```python
from build123d import *

# Parameters (mm, degrees)
SKETCH2_W           = 292
SKETCH2_H           = 160
BOSS_EXTRUDE1_DEPTH = 3
BOSS_EXTRUDE2_DEPTH = 3
BOSS_EXTRUDE3_START = -35
BOSS_EXTRUDE3_DEPTH = 55
SKETCH5_R           = 1.9
BOSS_EXTRUDE4_DEPTH = 5
BOSS_EXTRUDE5_START = 35
BOSS_EXTRUDE5_DEPTH = 35
SKETCH5_5_R         = 1.9
CUT_EXTRUDE1_DEPTH  = 309.76121842
SKETCH6_R           = 1.9
SKETCH6_W           = 6.2
SKETCH6_H           = 14.6
CUT_EXTRUDE2_DEPTH  = 225.15461182
SKETCH7_R           = 1.75
CUT_EXTRUDE3_DEPTH  = 225.15461182
BOSS_EXTRUDE6_DEPTH = 3
BOSS_EXTRUDE7_DEPTH = 21
SKETCH8_3_W         = 32
SKETCH8_3_H         = 38
CUT_EXTRUDE4_DEPTH  = 221.209195993


with BuildPart() as part:
    # Sketch2 → Boss-Extrude1 (new body)
    with BuildSketch(Plane(origin=(0, 0, 0), x_dir=(1, 0, 0), z_dir=(0, 1, 0))):
        with Locations((0, 80)):
            Rectangle(SKETCH2_W, SKETCH2_H)
    extrude(amount=BOSS_EXTRUDE1_DEPTH)

    # Sketch3 → Boss-Extrude2 (add)
    with BuildSketch(Plane(origin=(0, 3, 0), x_dir=(1, 0, 0), z_dir=(0, 1, 0))):
        with BuildLine():
            ThreePointArc((-49.25, -30.5), (-40.316756826, -8.933243174), (-18.75, 0))
            Line((-18.75, 0), (-146, 0))
            Line((-146, 0), (-146, -30.5))
            Line((-146, -30.5), (-49.25, -30.5))
        make_face()
        with BuildLine():
            Line((146, -30.5), (146, 0))
            Line((146, 0), (18.75, 0))
            ThreePointArc((18.75, 0), (40.316756826, -8.933243174), (49.25, -30.5))
            Line((49.25, -30.5), (146, -30.5))
        make_face()
    extrude(amount=-BOSS_EXTRUDE2_DEPTH)

    # Sketch4 → Boss-Extrude3 (add)
    with BuildSketch(Plane(origin=(146, 0, 0), x_dir=(0, 0, -1), z_dir=(1, 0, 0)).offset(BOSS_EXTRUDE3_START)):
        with BuildLine():
            Line((10.8, 21.7), (10.8, 3))
            Line((10.8, 3), (32.499999845, 3))
            ThreePointArc((32.499999845, 3), (19.277103137, 8.477103246), (13.8, 21.7))
            Line((13.8, 21.7), (10.8, 21.7))
        make_face()
        with BuildLine():
            ThreePointArc((51.2, 21.7), (45.722896754, 8.477103137), (32.499999845, 3))
            Line((32.499999845, 3), (54.2, 3))
            Line((54.2, 3), (54.2, 21.7))
            Line((54.2, 21.7), (51.2, 21.7))
        make_face()
    boss_extrude3 = extrude(amount=-BOSS_EXTRUDE3_DEPTH)

    # Sketch5 → Boss-Extrude4 (add)
    # profile 1 of 3: a face of its own
    with BuildSketch(Plane(origin=(111, 0, 0), x_dir=(0, 0, -1), z_dir=(1, 0, 0))):
        with BuildLine():
            Line((-4.5, 21.7), (-4.5, 0))
            Line((-4.5, 0), (69.5, 0))
            Line((69.5, 0), (69.5, 21.7))
            ThreePointArc((69.5, 21.7), (32.5, 58.7), (-4.5, 21.7))
        make_face()
        with Locations((24.875, 8.493112592)):
            Circle(SKETCH5_R, mode=Mode.SUBTRACT)
        with Locations((17.25, 21.7)):
            Circle(SKETCH5_R, mode=Mode.SUBTRACT)
        with Locations((40.125, 8.493112592)):
            Circle(SKETCH5_R, mode=Mode.SUBTRACT)
        with BuildLine():
            ThreePointArc((32.5, 3), (45.722896808, 8.477103192), (51.2, 21.7))
            Line((51.2, 21.7), (54.2, 21.7))
            Line((54.2, 21.7), (54.2, 3))
            Line((54.2, 3), (32.5, 3))
        make_face(mode=Mode.SUBTRACT)
        with BuildLine():
            ThreePointArc((26.3, 23.2), (32.5, 29.4), (38.7, 23.2))
            Line((38.7, 23.2), (38.7, 20.2))
            ThreePointArc((38.7, 20.2), (32.5, 14), (26.3, 20.2))
            Line((26.3, 20.2), (26.3, 23.2))
        make_face(mode=Mode.SUBTRACT)
        with Locations((47.75, 21.7)):
            Circle(SKETCH5_R, mode=Mode.SUBTRACT)
        with Locations((24.875, 34.906887408)):
            Circle(SKETCH5_R, mode=Mode.SUBTRACT)
        with Locations((40.125, 34.906887408)):
            Circle(SKETCH5_R, mode=Mode.SUBTRACT)
    # profile 2 of 3: a face of its own
    with BuildSketch(Plane(origin=(111, 0, 0), x_dir=(0, 0, -1), z_dir=(1, 0, 0))):
        with BuildLine():
            Line((-6.5, 0), (-4.5, 0))
            Line((-4.5, 0), (-4.5, 21.7))
            ThreePointArc((-4.5, 21.7), (32.5, 58.7), (69.5, 21.7))
            Line((69.5, 21.7), (69.5, 0))
            Line((69.5, 0), (71.5, 0))
            Line((71.5, 0), (71.5, 21.7))
            ThreePointArc((71.5, 21.7), (32.5, 60.7), (-6.5, 21.7))
            Line((-6.5, 21.7), (-6.5, 0))
        make_face()
    # profile 3 of 3: a face of its own
    with BuildSketch(Plane(origin=(111, 0, 0), x_dir=(0, 0, -1), z_dir=(1, 0, 0))):
        with BuildLine():
            Line((54.2, 21.7), (51.2, 21.7))
            ThreePointArc((51.2, 21.7), (45.722896808, 8.477103192), (32.5, 3))
            Line((32.5, 3), (54.2, 3))
            Line((54.2, 3), (54.2, 21.7))
        make_face()
    boss_extrude4 = extrude(amount=-BOSS_EXTRUDE4_DEPTH)

    # Sketch5<4> → Boss-Extrude5 (add)
    with BuildSketch(Plane(origin=(111, 0, 0), x_dir=(0, 0, -1), z_dir=(1, 0, 0)).offset(BOSS_EXTRUDE5_START)):
        with BuildLine():
            Line((-6.5, 0), (-4.5, 0))
            Line((-4.5, 0), (-4.5, 21.7))
            ThreePointArc((-4.5, 21.7), (32.5, 58.7), (69.5, 21.7))
            Line((69.5, 21.7), (69.5, 0))
            Line((69.5, 0), (71.5, 0))
            Line((71.5, 0), (71.5, 21.7))
            ThreePointArc((71.5, 21.7), (32.5, 60.7), (-6.5, 21.7))
            Line((-6.5, 21.7), (-6.5, 0))
        make_face()
    boss_extrude5 = extrude(amount=-BOSS_EXTRUDE5_DEPTH)

    # Sketch5<5> → Cut-Extrude1 (cut, through all)
    # profile 1 of 2: a face of its own
    with BuildSketch(Plane(origin=(111, 0, 0), x_dir=(0, 0, -1), z_dir=(1, 0, 0))):
        with BuildLine():
            Line((-4.5, 21.7), (-4.5, 0))
            Line((-4.5, 0), (69.5, 0))
            Line((69.5, 0), (69.5, 21.7))
            ThreePointArc((69.5, 21.7), (32.5, 58.7), (-4.5, 21.7))
        make_face()
        with Locations((24.875, 8.493112592)):
            Circle(SKETCH5_5_R, mode=Mode.SUBTRACT)
        with Locations((17.25, 21.7)):
            Circle(SKETCH5_5_R, mode=Mode.SUBTRACT)
        with Locations((40.125, 8.493112592)):
            Circle(SKETCH5_5_R, mode=Mode.SUBTRACT)
        with BuildLine():
            ThreePointArc((32.5, 3), (45.722896808, 8.477103192), (51.2, 21.7))
            Line((51.2, 21.7), (54.2, 21.7))
            Line((54.2, 21.7), (54.2, 3))
            Line((54.2, 3), (32.5, 3))
        make_face(mode=Mode.SUBTRACT)
        with BuildLine():
            ThreePointArc((26.3, 23.2), (32.5, 29.4), (38.7, 23.2))
            Line((38.7, 23.2), (38.7, 20.2))
            ThreePointArc((38.7, 20.2), (32.5, 14), (26.3, 20.2))
            Line((26.3, 20.2), (26.3, 23.2))
        make_face(mode=Mode.SUBTRACT)
        with Locations((47.75, 21.7)):
            Circle(SKETCH5_5_R, mode=Mode.SUBTRACT)
        with Locations((24.875, 34.906887408)):
            Circle(SKETCH5_5_R, mode=Mode.SUBTRACT)
        with Locations((40.125, 34.906887408)):
            Circle(SKETCH5_5_R, mode=Mode.SUBTRACT)
    # profile 2 of 2: a face of its own
    with BuildSketch(Plane(origin=(111, 0, 0), x_dir=(0, 0, -1), z_dir=(1, 0, 0))):
        with BuildLine():
            Line((54.2, 21.7), (51.2, 21.7))
            ThreePointArc((51.2, 21.7), (45.722896808, 8.477103192), (32.5, 3))
            Line((32.5, 3), (54.2, 3))
            Line((54.2, 3), (54.2, 21.7))
        make_face()
    cut_extrude1 = extrude(amount=CUT_EXTRUDE1_DEPTH, mode=Mode.SUBTRACT)

    # Sketch6 → Cut-Extrude2 (cut, through all)
    with BuildSketch(Plane(origin=(0, 3, 0), x_dir=(1, 0, 0), z_dir=(0, 1, 0))):
        with Locations(Location((120.3, -18.5, 0), (0, 0, 270))):
            Circle(SKETCH6_R)
        with Locations((140.9, -18.5)):
            Rectangle(SKETCH6_W, SKETCH6_H)
    cut_extrude2 = extrude(amount=-CUT_EXTRUDE2_DEPTH, mode=Mode.SUBTRACT)

    # Mirror1: Boss-Extrude3, Boss-Extrude4, Boss-Extrude5, Cut-Extrude1, Cut-Extrude2 across plane
    add(boss_extrude3.mirror(Plane(origin=(0, 0, 0), x_dir=(0, 0, 1), z_dir=(1, 0, 0))))
    add(boss_extrude4.mirror(Plane(origin=(0, 0, 0), x_dir=(0, 0, 1), z_dir=(1, 0, 0))))
    add(boss_extrude5.mirror(Plane(origin=(0, 0, 0), x_dir=(0, 0, 1), z_dir=(1, 0, 0))))
    add(cut_extrude1.mirror(Plane(origin=(0, 0, 0), x_dir=(0, 0, 1), z_dir=(1, 0, 0))), mode=Mode.SUBTRACT)
    add(cut_extrude2.mirror(Plane(origin=(0, 0, 0), x_dir=(0, 0, 1), z_dir=(1, 0, 0))), mode=Mode.SUBTRACT)

    # Sketch7 → Cut-Extrude3 (cut, through all)
    with BuildSketch(Plane(origin=(0, 3, 0), x_dir=(1, 0, 0), z_dir=(0, 1, 0))):
        with Locations(Location((-18, 14.5, 0), (0, 0, 270))):
            Circle(SKETCH7_R)
        with Locations(Location((18, 14.5, 0), (0, 0, 270))):
            Circle(SKETCH7_R)
        with Locations(Location((18, 50.5, 0), (0, 0, 270))):
            Circle(SKETCH7_R)
        with Locations(Location((-18, 50.5, 0), (0, 0, 270))):
            Circle(SKETCH7_R)
    extrude(amount=-CUT_EXTRUDE3_DEPTH, mode=Mode.SUBTRACT)



with BuildPart() as body_2:
    # Sketch8 → Boss-Extrude6 (new body)
    with BuildSketch(Plane(origin=(0, 21, 0), x_dir=(1, 0, 0), z_dir=(0, 1, 0))):
        with BuildLine():
            Line((-35, 141), (-35, 160))
            Line((-35, 160), (35, 160))
            Line((35, 160), (35, 141))
            ThreePointArc((35, 141), (0, 106), (-35, 141))
        make_face()
    extrude(amount=BOSS_EXTRUDE6_DEPTH)


with BuildPart() as part_1:
    add(part.part)

    add(body_2.part)  # Boss-Extrude7 merges body 2
    # Sketch10 → Boss-Extrude7 (add)
    with BuildSketch(Plane(origin=(0, 24, 0), x_dir=(1, 0, 0), z_dir=(0, 1, 0))):
        with BuildLine():
            Line((-38, 160), (-38, 141))
            ThreePointArc((-38, 141), (0, 103), (38, 141))
            Line((38, 141), (38, 160))
            Line((38, 160), (35, 160))
            Line((35, 160), (35, 141))
            ThreePointArc((35, 141), (0, 106), (-35, 141))
            Line((-35, 141), (-35, 160))
            Line((-35, 160), (-38, 160))
        make_face()
    extrude(amount=-BOSS_EXTRUDE7_DEPTH)

    # Sketch8<3> → Cut-Extrude4 (cut, through all)
    with BuildSketch(Plane(origin=(0, 21, 0), x_dir=(1, 0, 0), z_dir=(0, 1, 0))):
        with Locations((0, 141)):
            Rectangle(SKETCH8_3_W, SKETCH8_3_H)
        with BuildLine():
            Line((-16, 122), (-16, 160))
            Line((-16, 160), (-35, 160))
            Line((-35, 160), (-35, 141))
            ThreePointArc((-35, 141), (0, 106), (35, 141))
            Line((35, 141), (35, 160))
            Line((35, 160), (16, 160))
            Line((16, 160), (16, 122))
            Line((16, 122), (-16, 122))
        make_face()
    extrude(amount=-CUT_EXTRUDE4_DEPTH, mode=Mode.SUBTRACT)


solid = part_1.part
```
The model under review builds one solid part; all positions refer to its coordinate system, in mm. A direction names the side the tool comes from. Give positions to 0.01 mm unless a question says otherwise; leave off trailing zeros. Order: outer loops, then holes, each group sorted by start corner. A loop starts at its lowest first (then second) coordinate and runs counter-clockwise, first axis right, second up. Notation, with made-up numbers: (76, 88) - (102, 88) arc R18 cw to (102, 96) - close; hole circle Ø9 at (20, -33). An arc over 180 degrees is marked (long way). Use CSV: the item, a comma, the result in double quotes. Start each with the question number.
Q1. The part is to be moulded in two halves that separate along Y. For faces 4 (the flat face through (-128, 11, 4.5)), 5 (the cylindrical face through (126.28, 60.69, -33.36)), 6 (the cylindrical face through (-108.5, 14, -32.6)), say which applies: +Y half, -Y half, draft (parallel to the pull), parting line (faces both ways), or undercut.
Q2. Clearance check with flat-ended pins moving along their axes: pin 1 Ø9.5 at (y, z) = (12, -46) entering from +X; pin 2 Ø10 at (x, z) = (-88, -0.5) entering from +Y; pin 3 Ø1.5 at (x, z) = (74.5, -13) entering from +Y; pin 4 Ø8 at (x, y) = (-25.5, 24.5) entering from -Z. State where each tip first meets the part, or that it passes through.
Q3. We need section B-B, the plane z = -130. Write out the cut boundary in (x, y).
Q4. We need section A-A, the plane x = -100. Write out the cut boundary in (y, z).
Q5. We need section D-D, the plane x = 43. Write out the cut boundary in (y, z), and give its area (3 significant figures).
Q6. We need section C-C, the plane x = 0. Write out the cut boundary in (y, z), and give its area (3 significant figures).
Q7. To check wall thickness, follow line 1 along X through (y, z) = (37.5, -40.5); line 2 along Z through (x, y) = (-121, 15.5); line 3 along X through (y, z) = (2, 18). State the ranges of each line that lie inside material, in increasing order. Write a range as [from, to].
Q8. Tool access review of faces 1 (the flat face through (-111, 30, -32)), 2 (the flat face through (81, 12, -10.8)), 3 (the flat face through (-126, 12, 6.5)): name each direction out of +Z, -Z, +X, -X, +Y, -Y from which nothing blocks a thin tool from reaching the whole face with its end or side.
Outcome:
1,face 4,"draft"
1,face 5,"+Y half"
1,face 6,"undercut"
2,pin 1,"stops at x = 111"
2,pin 2,"stops at y = 3"
2,pin 3,"stops at y = 21.7"
2,pin 4,"stops at z = -160"
3,outline,"(-146, 0) - (-33.23, 0) - (-33.23, 21) - (33.23, 21) - (33.23, 0) - (146, 0) - (146, 3) - (36.37, 3) - (36.37, 24) - (-36.37, 24) - (-36.37, 3) - (-146, 3) - close"
4,outline,"(0, -160) - (3, -160) - (3, -54.2) - (21.7, -54.2) - (21.7, -51.2) arc R18.7 cw to (21.7, -13.8) - (21.7, -10.8) - (3, -10.8) - (3, 30.5) - (0, 30.5) - close"
5,outline,"(0, -160) - (3, -160) - (3, 12) - (0, 12) - close"
5,area,"516 mm^2"
6,outline,"(0, -106) - (21, -106) - (21, -160) - (24, -160) - (24, -103) - (3, -103) - (3, 0) - (0, 0) - close"
6,area,"543 mm^2"
7,line 1,"x = [-111, -106], [106, 111]"
7,line 2,"z = [-71.5, -69.5], [4.5, 6.5]"
7,line 3,"x = [-146, -144], [-137.8, -122.13], [-118.47, -46.57], [46.57, 118.47], [122.13, 137.8], [144, 146]"
8,face 1,"-X, -Y"
8,face 2,"+Z, +Y"
8,face 3,"+Z, +X, -X, +Y"
